Work out the finished part from the listing and answer in its coordinate system (mm). A direction names the side the tool comes from. Coordinates: 2 decimals unless noted, no trailing zeros. Order: outer loops, then holes, each group sorted by start corner. A loop starts at its lowest first (then second) coordinate and runs counter-clockwise, first axis right, second up. Notation, with made-up numbers: (89, -22.5) -> (111, -22.5) arc R13 ccw to (111, -2.5) -> close; hole circle Ø10 at (0, 77). An arc over 180 degrees is marked (long way). Write item = value, one per line. Start each with the question number.
Q1. The part is cut by section A-A, the plane x = 22.75. Determine the outline of the cut face in (y, z), plus the area to 3 significant figures.
Q2. The part is cut by section C-C, the plane z = 19.5. Determine the outline of the cut face in (x, y).
Q3. Flat-ended cylindrical pins translate along their axes: pin 1 (5 mm diameter, centred on x = 8, y = 46, fed in from -Z); pin 2 (1 mm diameter, centred on x = 5, z = 12, fed in from +Y); pin 3 (10 mm diameter, centred on x = 4.5, z = -15.5, fed in from +Y). Find the tip coordinate at first contact, or state that the pin passes through.
Q4. For a pull along X with two mould halves and no side action, classify faces 4 (the flat face through (13, 4, -87.25)), 5 (the flat face through (27, 32, 2)), 6 (the flat face through (13, 5, -124.5)) as +X half, -X half, draft (parallel to the pull), parting line (faces both ways), or undercut.
Q5. Which of the six approach directions +Z, -Z, +X, -X, +Y, -Y give full straight-line access (tool end or side, diameter ignored) to faces 1 (the flat face through (1, 0, -104)), 2 (the flat face through (13, 6, -84.5)), 3 (the flat face through (1.75, 4, -105))?
Q6. The part is cut by section D-D, the plane y = 35.5. Determine the outline of the cut face in (x, z).
Q7. The part is cut by section B-B, the plane y = 22.5. Determine the outline of the cut face in (x, z), plus the area to 3 significant figures.
Q8. Straight lines are drawn through the part: L1, parallel to Z at x = 17.5, y = 5; L2, parallel to X at y = 4.5, z = 110; L3, parallel to Z at x = 15.5, y = 11. For each, find the intervals that lie inside material, in ascending order. Write a range as from..to.
```python
from build123d import *

# Parameters (mm, degrees)
BOSS_EXTRUDE1_DEPTH = 27
SKETCH3_W           = 23.5
SKETCH3_H           = 34.5
CUT_EXTRUDE1_DEPTH  = 7.5


with BuildPart() as part:
    # Sketch1 → Boss-Extrude1 (new body)
    with BuildSketch(Plane(origin=(0, 0, 0), x_dir=(0, 0, -1), z_dir=(1, 0, 0))):
        with BuildLine():
            Line((-124.5, 0), (-84.5, 0))
            Line((-84.5, 0), (-84.5, 12))
            ThreePointArc((-84.5, 12), (0, 30.7274152), (84.5, 12))
            Line((84.5, 12), (84.5, 0))
            Line((84.5, 0), (124.5, 0))
            Line((124.5, 0), (124.5, 10))
            ThreePointArc((124.5, 10), (0, 62.423059842), (-124.5, 10))
            Line((-124.5, 10), (-124.5, 0))
        make_face()
    extrude(amount=BOSS_EXTRUDE1_DEPTH)

    # Sketch3 → Cut-Extrude1 (cut)
    with BuildSketch(Plane.XZ):
        with Locations((13.5, 102.98)):
            Rectangle(SKETCH3_W, SKETCH3_H)
        with Locations((13.5, -104.5)):
            Rectangle(SKETCH3_W, SKETCH3_H)
    extrude(amount=-CUT_EXTRUDE1_DEPTH, mode=Mode.SUBTRACT)


solid = part.part
```
Model answer:
q1.outline = (0, -124.5) -> (10, -124.5) arc R174.05 ccw to (10, 124.5) -> (0, 124.5) -> (0, 120.23) -> (7.5, 120.23) -> (7.5, 85.73) -> (0, 85.73) -> (0, 84.5) -> (12, 84.5) arc R200 cw to (12, -84.5) -> (0, -84.5) -> (0, -87.25) -> (7.5, -87.25) -> (7.5, -121.75) -> (0, -121.75) -> close
q1.area = 6,820 mm2
q2.outline = (0, 29.77) -> (27, 29.77) -> (27, 61.33) -> (0, 61.33) -> close
q3.pin_1 = -78.92
q3.pin_2 = 62.04
q3.pin_3 = 62.11
q4.face_4 = undercut
q4.face_5 = +X half
q4.face_6 = draft
q5.face_1 = +Z, -Z, +X, -X, -Y
q5.face_2 = +X, -X, -Y
q5.face_3 = -Y
q6.outline = (0, -92.99) -> (27, -92.99) -> (27, 92.99) -> (0, 92.99) -> close
q7.outline = (0, -110.92) -> (27, -110.92) -> (27, -56.77) -> (0, -56.77) -> close; (0, 56.77) -> (27, 56.77) -> (27, 110.92) -> (0, 110.92) -> close
q7.area = 2,920 mm2
q8.L1 = -124.5..-121.75, -87.25..-84.5, 84.5..85.73, 120.23..124.5
q8.L2 = 0..1.75, 25.25..27
q8.L3 = -123.52..-84.5, 84.5..123.52
